Input: part model. Units: mm. Frame: model coordinates. Face numbers are marked on the shaded views. A direction names the side the tool comes from. Round coordinates to 2 decimals unless told otherwise and drop trailing zeros. Loops run counter-clockwise (first coordinate to the right, second up) from the corner with the lowest first, then second, coordinate; pieces in that order, holes last. Notation, with made-up numbers: (73.25, 87) - (112.25, 87) arc R22 ccw to (112.25, 118) - close; hole circle Ø6 at (83.5, -31.5). An arc over 180 degrees is marked (long way). One line per question, with ' | ' between items. Start each with the question number.
Autodesk Inventor part; units mm, degrees
ref_plane "YZ Plane" through (0, 0, 0) normal (1, 0, 0) x (0, 1, 0)
ref_plane "XZ Plane" through (0, 0, 0) normal (0, 1, 0) x (-1, 0, 0)
ref_plane "XY Plane" through (0, 0, 0) normal (0, 0, 1) x (1, 0, 0)
sketch "スケッチ1" plane through (0, 0, 0) normal (0, 0, 1) x (1, 0, 0)
  circle A0 centre (0, 0) radius 3
  circle A1 centre (0, 0) radius 5
  dimension "d0" = 6
  dimension "d1" = 10
extrude "押し出し1" add sketch "スケッチ1" along normal blind 3
sketch "スケッチ2" plane through (0, 0, 0) normal (0, 0, -1) x (-1, 0, 0)
  circle A0 centre (0, 0) radius 3
  circle A1 centre (0, 0) radius 5
  circle A2 centre (0, 0) radius 5.6
  dimension "d4" = 11.2
extrude "押し出し2" add sketch "スケッチ2" against normal blind 0.6 contours A2
sketch "スケッチ3" plane through (0, 0, 3) normal (0, 0, 1) x (1, 0, 0)
  circle A0 centre (0, 0) radius 3
  circle A1 centre (0, 0) radius 5
  circle A2 centre (0, 0) radius 4.5
  circle A3 centre (0, 0) radius 3.5
  dimension "d7" = 0.5
  dimension "d8" = 0.5
extrude "押し出し3" cut sketch "スケッチ3" against normal blind 0.5 contours A2
sketch "スケッチ4" plane through (0, 0, 0) normal (0, 0, -1) x (-1, 0, 0)
  circle A0 centre (0, 0) radius 3.5
  circle A1 centre (0, 0) radius 4.5
extrude "押し出し4" cut sketch "スケッチ4" against normal blind 0.5
sketch "スケッチ5" plane through (0, 0, 0) normal (0, 0, -1) x (-1, 0, 0)
  point P0 (0, 0)
sketch "スケッチ6" plane through (0, 0, 0.6) normal (0, 0, 1) x (1, 0, 0)
  circle A0 centre (0, 0) radius 5
  circle A1 centre (0, 0) radius 5.6
  dimension "d13" = 10
  dimension "d14" = 0.6
extrude "押し出し5" cut sketch "スケッチ6" against normal blind 0.6
properties part number "ベアリングHd6-D10-B3F無し甲" material "鋼、炭素鋼"
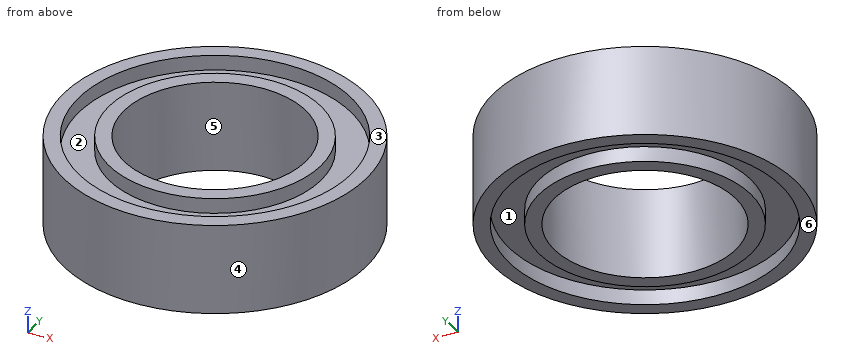
(1) Pull-direction query (X, two-part tool) for the marked faces 4, 5 and 6; classes: released by +X, released by -X, zero draft, split by the parting line, or undercut.
(2) Line query: line 1 along Y through (x, z) = (0, 0.25); line 2 along Y through (x, z) = (0, 1.3); line 3 along X through (y, z) = (-4, 0.1). Output: solid intervals per line, ascending. Write a range as from..to.
(3) Section D-D, the plane z = 0.65. Output: boundary loops of the cut face in (x, y), plus the area to 3 significant figures.
(4) Reachability of the marked faces 1, 2 and 3 from +Z, -Z, +X, -X, +Y, -Y: full face, straight path, thin tool, end or side. Return the list, or none.
(5) Pin query (flat end, axial travel): P1, Ø1.5, axis at y = -2.5, z = 1.5, coming from the +X side; P2, Ø1, axis at y = 1, z = 1, coming from the -X side. Return the tip coordinate at first contact, or that it passes through.
(6) Section C-C, the plane y = 3.75. Output: boundary loops of the cut face in (x, z), plus the area to 3 significant figures.
(7) Section A-A, the plane x = 0. Output: boundary loops of the cut face in (y, z), plus the area to 3 significant figures.
Derived:
1) face 4: split by the parting line | face 5: undercut | face 6: zero draft
2) line 1: y = -5..-4.5, -3.5..-3, 3..3.5, 4.5..5 | line 2: y = -5..-3, 3..5 | line 3: x = -3..-2.06, 2.06..3
3) outline: circle Ø10 at (0, 0); hole circle Ø6 at (0, 0) | area: 50.3 mm²
4) face 1: -Z | face 2: +Z | face 3: +Z, +X, -X, +Y, -Y
5) P1: stops at x = 4.68 | P2: stops at x = -4.97
6) outline: (-3.31, 0) - (-2.49, 0) - (-2.49, 0.5) - (2.49, 0.5) - (2.49, 0) - (3.31, 0) - (3.31, 3) - (2.49, 3) - (2.49, 2.5) - (-2.49, 2.5) - (-2.49, 3) - (-3.31, 3) - close | area: 14.9 mm²
7) outline: (-5, 0) - (-4.5, 0) - (-4.5, 0.5) - (-3.5, 0.5) - (-3.5, 0) - (-3, 0) - (-3, 3) - (-3.5, 3) - (-3.5, 2.5) - (-4.5, 2.5) - (-4.5, 3) - (-5, 3) - close; (3, 0) - (3.5, 0) - (3.5, 0.5) - (4.5, 0.5) - (4.5, 0) - (5, 0) - (5, 3) - (4.5, 3) - (4.5, 2.5) - (3.5, 2.5) - (3.5, 3) - (3, 3) - close | area: 10.0 mm²
